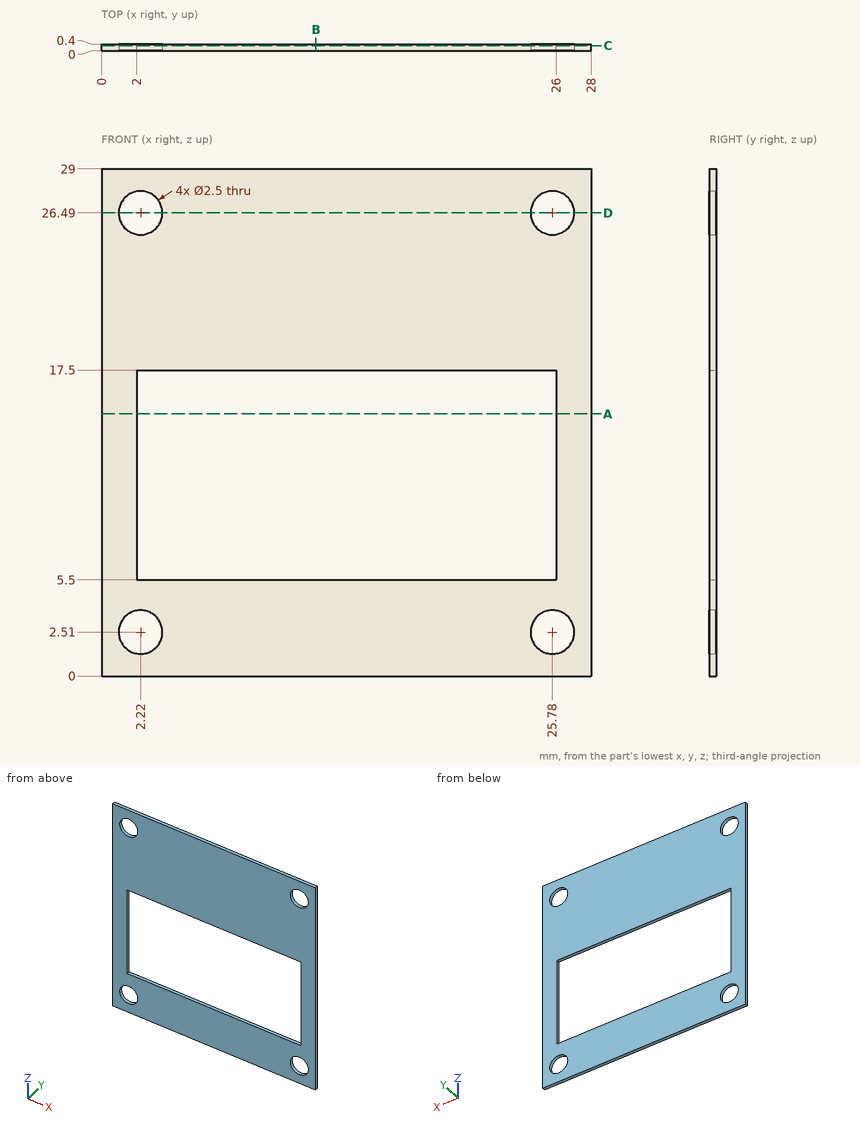
Part print with two shaded views. Sizes in mm from the minimum x, y, z corner. Give positions to 0.01 mm unless a question says otherwise; leave off trailing zeros. Order: outer loops, then holes, each group sorted by start corner. A loop starts at its lowest first (then second) coordinate and runs counter-clockwise, first axis right, second up. Notation, with made-up numbers: M 38,43.25 L 46,43.25 A15 ccw 46,70.25 Z; hole C -15,25 d7. An arc over 180 degrees is marked long. Put each result on its own line as item: value.
Item 1: Cut at C-C on y = 0.3. Write the cut outline in (x, z), then the cut area to 3 significant figures.
Results are:
outline: M 0,0 L 28,0 L 28,29 L 0,29 Z; hole C 2.22,2.51 d2.5; hole C 2.22,26.49 d2.5; hole M 2,5.5 L 26,5.5 L 26,17.5 L 2,17.5 Z; hole C 25.78,2.51 d2.5; hole C 25.78,26.49 d2.5
area: 504 mm2
Item 2: Cut at B-B on x = 12.25. Write the cut outline in (y, z).
Results are:
outline: M 0,0 L 0.4,0 L 0.4,5.5 L 0,5.5 Z; M 0,17.5 L 0.4,17.5 L 0.4,29 L 0,29 Z
Item 3: Cut at D-D on z = 26.49. Write the cut outline in (x, y).
Results are:
outline: M 0,0 L 0.97,0 L 0.97,0.4 L 0,0.4 Z; M 3.47,0 L 24.53,0 L 24.53,0.4 L 3.47,0.4 Z; M 27.03,0 L 28,0 L 28,0.4 L 27.03,0.4 Z
Item 4: Wall check: probe 1 along X at (y, z) = (0.2, 26.5); probe 2 along Z at (x, y) = (5, 0.15); probe 3 along X at (y, z) = (0.1, 15). Give the ranges that are in metal, low to high.
Results are:
probe 1: 0 to 0.97, 3.47 to 24.53, 27.03 to 28
probe 2: 0 to 5.5, 17.5 to 29
probe 3: 0 to 2, 26 to 28
Item 5: Drop flat-ended pins along their axis: pin 1 Ø4 at (x, z) = (2.22, 26.49) entering from -Y; pin 2 Ø2 at (x, z) = (2.22, 2.51) entering from +Y. Give the stop position or say it passes through.
Results are:
pin 1: y = 0
pin 2: through
Item 6: Cut at A-A on z = 15. Write the cut outline in (x, y), then the cut area to 3 significant figures.
Results are:
outline: M 0,0 L 2,0 L 2,0.4 L 0,0.4 Z; M 26,0 L 28,0 L 28,0.4 L 26,0.4 Z
area: 1.60 mm2
